```python
from build123d import *

# Parameters (mm, degrees)
SKETCH1_W                  = 25.4
SKETCH1_H                  = 1498.6
BOSS_EXTRUDE1_DEPTH        = 25.4
SKETCH2_W                  = 23.114
SKETCH2_H                  = 23.114
CUT_EXTRUDE1_DEPTH         = 1499.6
M3_5_CLEARANCE_HOLE1_D     = 4.1402
M3_5_CLEARANCE_HOLE1_DEPTH = 25.4
M3_5_CLEARANCE_HOLE2_D     = 4.1402
M3_5_CLEARANCE_HOLE2_DEPTH = 25.4
CHAMFER1_SIZE              = 2.159
FILLET1_R                  = 0.8128
FILLET2_R                  = 3.0988
SKETCH8_W                  = 95.882963774
SKETCH8_H                  = 79.338329604
CUT_EXTRUDE3_DEPTH         = 1397
SKETCH9_W                  = 55.647897921
SKETCH9_H                  = 59.659370493
CUT_EXTRUDE4_DEPTH         = 2.286
SKETCH10_W                 = 60.180202688
SKETCH10_H                 = 53.53268885
CUT_EXTRUDE5_DEPTH         = 2.286


with BuildPart() as part:
    # Sketch1 → Boss-Extrude1 (new body)
    with BuildSketch(Plane(origin=(0, 0, 0), x_dir=(0, -1, 0), z_dir=(-1, 0, 0))):
        with Locations((-12.7, 0)):
            Rectangle(SKETCH1_W, SKETCH1_H)
    extrude(amount=-BOSS_EXTRUDE1_DEPTH)

    # Sketch2 → Cut-Extrude1 (cut, through all)
    with BuildSketch(Plane(origin=(0, 0, -749.3), x_dir=(-1, 0, 0), z_dir=(0, 0, -1))):
        with Locations((-13.843, 13.843)):
            Rectangle(SKETCH2_W, SKETCH2_H)
    extrude(amount=-CUT_EXTRUDE1_DEPTH, mode=Mode.SUBTRACT)

    # M3.5 Clearance Hole1
    with Locations(Plane(origin=(0, 0, 0), x_dir=(-1, 0, 0), z_dir=(0, -1, 0))):
        with Locations((-12.7, 736.6), (-12.7, 711.2), (-12.7, 685.8), (-12.7, 660.4), (-12.7, 635), (-12.7, 609.6), (-12.7, 584.2), (-12.7, 558.8), (-12.7, 533.4), (-12.7, 508), (-12.7, 482.6), (-12.7, 457.2), (-12.7, 431.8), (-12.7, 406.4), (-12.7, 381), (-12.7, 355.6), (-12.7, 330.2), (-12.7, 304.8), (-12.7, 279.4), (-12.7, 254), (-12.7, 228.6), (-12.7, 203.2), (-12.7, 177.8), (-12.7, 152.4), (-12.7, 127), (-12.7, 101.6), (-12.7, 76.2), (-12.7, 50.8), (-12.7, 25.4), (-12.7, 0), (-12.7, -25.4), (-12.7, -50.8), (-12.7, -76.2), (-12.7, -101.6), (-12.7, -127), (-12.7, -152.4), (-12.7, -177.8), (-12.7, -203.2), (-12.7, -228.6), (-12.7, -254), (-12.7, -279.4), (-12.7, -304.8), (-12.7, -330.2), (-12.7, -355.6), (-12.7, -381), (-12.7, -406.4), (-12.7, -431.8), (-12.7, -457.2), (-12.7, -482.6), (-12.7, -508), (-12.7, -533.4), (-12.7, -558.8), (-12.7, -584.2), (-12.7, -609.6), (-12.7, -635), (-12.7, -660.4), (-12.7, -685.8), (-12.7, -711.2), (-12.7, -736.6)):
            Hole(M3_5_CLEARANCE_HOLE1_D / 2, depth=M3_5_CLEARANCE_HOLE1_DEPTH)

    # M3.5 Clearance Hole2
    with Locations(Plane.ZY):
        with Locations((711.2, 12.7), (736.6, 12.7), (685.8, 12.7), (660.4, 12.7), (635, 12.7), (609.6, 12.7), (584.2, 12.7), (558.8, 12.7), (533.4, 12.7), (508, 12.7), (482.6, 12.7), (457.2, 12.7), (431.8, 12.7), (406.4, 12.7), (381, 12.7), (355.6, 12.7), (330.2, 12.7), (304.8, 12.7), (279.4, 12.7), (254, 12.7), (228.6, 12.7), (203.2, 12.7), (177.8, 12.7), (152.4, 12.7), (127, 12.7), (101.6, 12.7), (76.2, 12.7), (50.8, 12.7), (25.4, 12.7), (0, 12.7), (-25.4, 12.7), (-50.8, 12.7), (-76.2, 12.7), (-101.6, 12.7), (-127, 12.7), (-152.4, 12.7), (-177.8, 12.7), (-203.2, 12.7), (-228.6, 12.7), (-254, 12.7), (-279.4, 12.7), (-304.8, 12.7), (-330.2, 12.7), (-355.6, 12.7), (-381, 12.7), (-406.4, 12.7), (-431.8, 12.7), (-457.2, 12.7), (-482.6, 12.7), (-508, 12.7), (-533.4, 12.7), (-558.8, 12.7), (-584.2, 12.7), (-609.6, 12.7), (-635, 12.7), (-660.4, 12.7), (-685.8, 12.7), (-711.2, 12.7), (-736.6, 12.7)):
            Hole(M3_5_CLEARANCE_HOLE2_D / 2, depth=M3_5_CLEARANCE_HOLE2_DEPTH)

    # Chamfer1
    chamfer1_edges = [part.edges().sort_by_distance(p)[0] for p in [
        (25.4, 1.143, -749.3),
        (1.143, 25.4, 749.3),
        (1.143, 25.4, -749.3),
        (25.4, 1.143, 749.3),
    ]]
    chamfer(chamfer1_edges, length=CHAMFER1_SIZE)

    # Fillet1
    fillet1_edges = [part.edges().sort_by_distance(p)[0] for p in [
        (2.286, 2.286, 0),
    ]]
    fillet(fillet1_edges, radius=FILLET1_R)

    # Fillet2
    fillet2_edges = [part.edges().sort_by_distance(p)[0] for p in [
        (0, 0, 0),
    ]]
    fillet(fillet2_edges, radius=FILLET2_R)

    # Sketch8 → Cut-Extrude3 (cut)
    with BuildSketch(Plane.XY.offset(749.3)):
        with Locations((2.286, 3.0988)):
            Rectangle(SKETCH8_W, SKETCH8_H)
    extrude(amount=-CUT_EXTRUDE3_DEPTH, mode=Mode.SUBTRACT)

    # Sketch9 → Cut-Extrude4 (cut)
    with BuildSketch(Plane.XY.offset(-647.7)):
        with Locations((1.567971806, 1.525578147)):
            Rectangle(SKETCH9_W, SKETCH9_H)
    extrude(amount=-CUT_EXTRUDE4_DEPTH, mode=Mode.SUBTRACT)

    # Sketch10 → Cut-Extrude5 (cut)
    with BuildSketch(Plane(origin=(0, 0, -749.3), x_dir=(-1, 0, 0), z_dir=(0, 0, -1))):
        with Locations((-0.996649486, 3.303060092)):
            Rectangle(SKETCH10_W, SKETCH10_H)
    extrude(amount=-CUT_EXTRUDE5_DEPTH, mode=Mode.SUBTRACT)


solid = part.part
```
CAD build for the part. Positions are in the model's coordinates, mm. A direction names the side the tool comes from. Coordinates: 2 decimals unless noted, no trailing zeros. Write each loop counter-clockwise with the first axis right and the second up, starting at its lowest first coordinate (ties: lowest second). Pieces come first, ordered by that corner, then holes.
(1) 3-axis set-ups, long thin cutter, end or side, ignore diameter. For faces 1 (the face through (2.286, 14, -699)), 2 (the face through (12.431, 1.159, -662.452)): which of +Z, -Z, +X, -X, +Y, -Y reach the whole face in a straight line?
(2) Cut at B-B, the plane y = 12.7. List the corners of the cut face in (x, z), and give its area (3 significant figures).
(3) Drill centre lines: probe 1 along Z at (x, y) = (12.7, 1.1); probe 2 along Y at (x, z) = (14, -700). Where is each one in solid material? Low to high.
(4) Cut at A-A, the plane z = -736.6. List the corners of the cut face in (x, y).
(5) Flat gauge pins, fed straight in: pin 1 (5.5 mm diameter, centred on y = 12.7, z = -736.6, fed in from +X); pin 2 (3.5 mm diameter, centred on x = 12.7, z = -685.8, fed in from +Y); pin 3 (6.5 mm diameter, centred on x = 19, z = -704.5, fed in from +Y). Where does each tip first touch, or does it go through?
(6) Two-plate mould, pull along Z, no slides. Class faces 3 (the face through (1, 7, -649.986)), 4 (the face through (14, 2.286, -699)), 5 (the face through (1.16, 12.79, -734.53)), 6 (the face through (12.431, 1.159, -713.252)): +Z half, -Z half, draft (parallel to the pull), parting line (faces both ways), or undercut.
(7) Cut at D-D, the plane z = -674. List the corners of the cut face in (x, y).
Geometry says:
1. face 1: +Z, -Z, +X, +Y
1. face 2: +Y, -Y
2. outline: (0, -747.01) - (2.29, -747.01) - (2.29, -738.67) - (0, -738.67) - close; (0, -734.53) - (2.29, -734.53) - (2.29, -713.27) - (0, -713.27) - close; (0, -709.13) - (2.29, -709.13) - (2.29, -687.87) - (0, -687.87) - close; (0, -683.73) - (2.29, -683.73) - (2.29, -662.47) - (0, -662.47) - close; (0, -658.33) - (2.29, -658.33) - (2.29, -649.99) - (0, -649.99) - close
2. area: 184 mm2
3. probe 1: z = -747.01 to -738.67, -734.53 to -713.27, -709.13 to -687.87, -683.73 to -662.47, -658.33 to -649.99
3. probe 2: y = 0 to 2.29
4. outline: (0, 3.1) arc R3.1 ccw to (3.1, 0) - (10.63, 0) - (10.63, 2.29) - (3.1, 2.29) arc R0.81 cw to (2.29, 3.1) - (2.29, 10.63) - (0, 10.63) - close; (0, 14.77) - (2.29, 14.77) - (2.29, 25.4) - (0, 25.4) - close; (14.77, 0) - (25.4, 0) - (25.4, 2.29) - (14.77, 2.29) - close
5. pin 1: stops at x = 2.29
5. pin 2: passes through
5. pin 3: stops at y = 2.29
6. face 3: +Z half
6. face 4: draft
6. face 5: undercut
6. face 6: undercut
7. outline: (0, 3.1) arc R3.1 ccw to (3.1, 0) - (25.4, 0) - (25.4, 2.29) - (3.1, 2.29) arc R0.81 cw to (2.29, 3.1) - (2.29, 25.4) - (0, 25.4) - close
